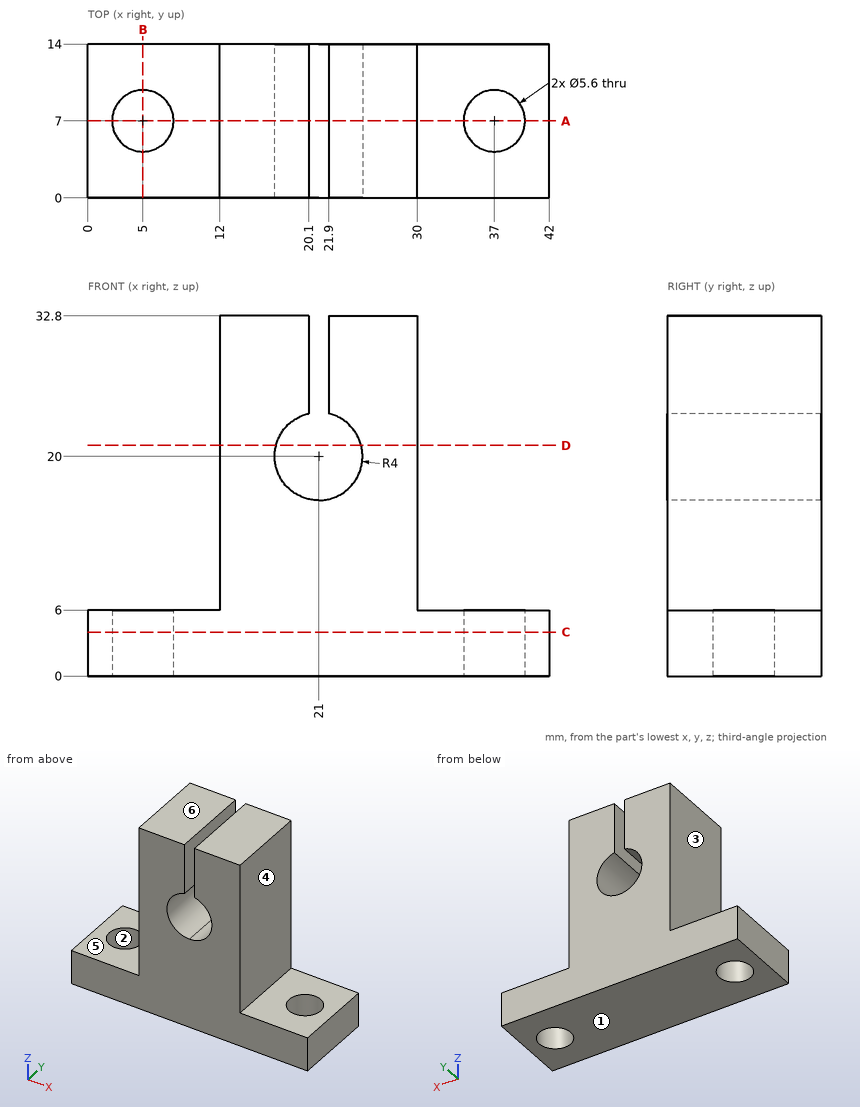
Job drawing, mm, ordinate dimensions from the low corner. One solid piece. A direction names the side the tool comes from. Give positions to 0.01 mm unless a question says otherwise; leave off trailing zeros. Order: outer loops, then holes, each group sorted by start corner. A loop starts at its lowest first (then second) coordinate and runs counter-clockwise, first axis right, second up. Notation, with made-up numbers: M -38,24 L -2,24 A30 ccw -2,53 Z; hole C 22,28 d6. An arc over 180 degrees is marked long. Return JSON: item names as keys, results as strings.
Q1. Two-plate mould, pull along X, no slides. Class the marked faces 1, 2 and 3: pulls with the +X half, pulls with the -X half, needs draft (parallel to the pull), parting line crosses it, or undercut.
Answer list:
{"face 1": "needs draft", "face 2": "undercut", "face 3": "pulls with the -X half"}
Q2. Wall check: probe 1 along X at (y, z) = (7, 2.05); probe 2 along Y at (x, z) = (37, 1); probe 3 along X at (y, z) = (5.5, 24). Give the ranges that are in metal, low to high. Write a range as from..to.
Answer list:
{"probe 1": "x = 0..2.2, 7.8..34.2, 39.8..42", "probe 2": "y = 0..4.2, 9.8..14", "probe 3": "x = 12..20.1, 21.9..30"}
Q3. Band-saw the part on B-B (x = 5). Give the cut face in (y, z).
Answer list:
{"outline": "M 0,0 L 4.2,0 L 4.2,6 L 0,6 Z; M 9.8,0 L 14,0 L 14,6 L 9.8,6 Z"}
Q4. Band-saw the part on A-A (y = 7). Give the cut face in (x, z).
Answer list:
{"outline": "M 0,0 L 2.2,0 L 2.2,6 L 0,6 Z; M 7.8,0 L 34.2,0 L 34.2,6 L 30,6 L 30,32.8 L 21.9,32.8 L 21.9,23.9 A4 cw long 20.1,23.9 L 20.1,32.8 L 12,32.8 L 12,6 L 7.8,6 Z; M 39.8,0 L 42,0 L 42,6 L 39.8,6 Z"}
Q5. 3-axis set-ups, long thin cutter, end or side, ignore diameter. For the marked faces 4, 5 and 6: which of +Z, -Z, +X, -X, +Y, -Y reach the whole face in a straight line?
Answer list:
{"face 4": "+Z, +X, +Y, -Y", "face 5": "+Z, -X, +Y, -Y", "face 6": "+Z, +X, -X, +Y, -Y"}
Q6. Band-saw the part on D-D (z = 21). Give the cut face in (x, y), then the cut area to 3 significant figures.
Answer list:
{"outline": "M 12,0 L 17.13,0 L 17.13,14 L 12,14 Z; M 24.87,0 L 30,0 L 30,14 L 24.87,14 Z", "area": "144 mm^2"}
Q7. Band-saw the part on C-C (z = 4). Give the cut face in (x, y), then the cut area to 3 significant figures.
Answer list:
{"outline": "M 0,0 L 42,0 L 42,14 L 0,14 Z; hole C 5,7 d5.6; hole C 37,7 d5.6", "area": "539 mm^2"}
Q8. Flat gauge pins, fed straight in: pin 1 (1.5 mm diameter, centred on y = 11.5, z = 11.5, fed in from -X); pin 2 (5 mm diameter, centred on y = 10, z = 29, fed in from +X); pin 3 (6 mm diameter, centred on x = 4, y = 3.5, fed in from +Z). Where does each tip first touch, or does it go through?
Answer list:
{"pin 1": "stops at x = 12", "pin 2": "stops at x = 30", "pin 3": "stops at z = 6"}
